Source: CAD feature listing. Evaluate the final solid. Frame: model axes, mm. Face numbers are marked on the shaded views. A direction names the side the tool comes from. Give positions to 0.01 mm unless a question says otherwise; leave off trailing zeros. Loops run counter-clockwise (first coordinate to the right, second up) from the corner with the lowest first, then second, coordinate; pieces in that order, holes last. Notation, with made-up numbers: M 79,14.5 L 136,14.5 A15 ccw 136,27.5 Z; hole C -21.5,54 d9. An arc over 180 degrees is marked long. Write item = value, one per line.
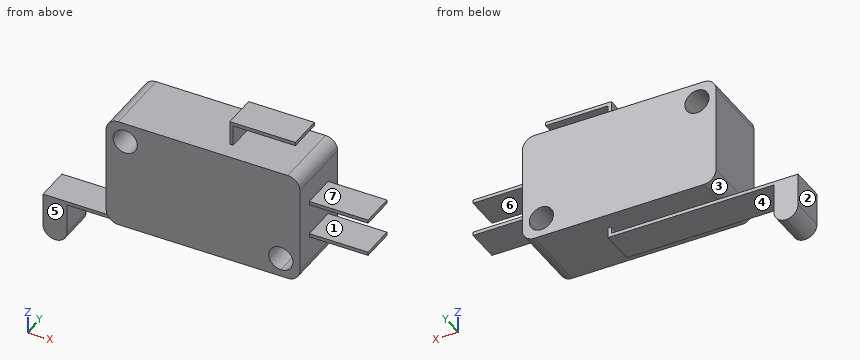
from build123d import *

# Parameters (mm, degrees)
SKETCH1_W           = 28
SKETCH1_H           = 16
BOSS_EXTRUDE1_DEPTH = 10
BOSS_EXTRUDE2_DEPTH = 1.5
SKETCH4_W           = 0.5
SKETCH4_H           = 5
BOSS_EXTRUDE3_DEPTH = 27
SKETCH6_W           = 3.5
SKETCH6_H           = 6
BOSS_EXTRUDE4_DEPTH = 5
FILLET1_R           = 1.75
BOSS_EXTRUDE5_DEPTH = 3.5
SKETCH8_W           = 0.5
SKETCH8_H           = 5
BOSS_EXTRUDE6_DEPTH = 9
BOSS_EXTRUDE7_DEPTH = 8.5
CUT_EXTRUDE1_DEPTH  = 45.547727215
CUT_EXTRUDE2_DEPTH  = 45.547727215
FILLET2_R           = 1.75


with BuildPart() as part:
    # Sketch1 → Boss-Extrude1 (new body)
    with BuildSketch(Plane(origin=(0, 0, 0), x_dir=(1, 0, 0), z_dir=(0, 1, 0))):
        with Locations((14, 8)):
            Rectangle(SKETCH1_W, SKETCH1_H)
    extrude(amount=BOSS_EXTRUDE1_DEPTH)

    # Sketch3 → Boss-Extrude2 (add)
    with BuildSketch(Plane(origin=(0, 0, -16), x_dir=(-1, 0, 0), z_dir=(0, 0, -1))):
        Polygon((-17, 2.5), (-17, 5), (-17, 7.5), (-16.5, 7.5), (-16.5, 2.5), align=None)
    extrude(amount=BOSS_EXTRUDE2_DEPTH)

    # Sketch4 → Boss-Extrude3 (add)
    with BuildSketch(Plane.ZY.offset(-16.5)):
        with Locations((-17.25, 5)):
            Rectangle(SKETCH4_W, SKETCH4_H)
    extrude(amount=BOSS_EXTRUDE3_DEPTH)

    # Sketch6 → Boss-Extrude4 (add)
    with BuildSketch(Plane.XZ.offset(-2.5)):
        with Locations((-8.75, -20.5)):
            Rectangle(SKETCH6_W, SKETCH6_H)
    extrude(amount=-BOSS_EXTRUDE4_DEPTH)

    # Fillet1
    fillet1_edges = [part.edges().sort_by_distance(p)[0] for p in [
        (-7, 5, -23.5),
        (-10.5, 5, -23.5),
    ]]
    fillet(fillet1_edges, radius=FILLET1_R - 0.0001)  # a hair under: the kernel refuses the full size

    # Sketch7 → Boss-Extrude5 (add)
    with BuildSketch(Plane.XY):
        Polygon((16.5, 2.5), (17, 2.5), (17, 5), (17, 7.5), (16.5, 7.5), align=None)
    extrude(amount=BOSS_EXTRUDE5_DEPTH)

    # Sketch8 → Boss-Extrude6 (add)
    with BuildSketch(Plane(origin=(17, 0, 0), x_dir=(0, 0, -1), z_dir=(1, 0, 0))):
        with Locations((-3.25, 5)):
            Rectangle(SKETCH8_W, SKETCH8_H)
    extrude(amount=BOSS_EXTRUDE6_DEPTH)

    # Sketch9 → Boss-Extrude7 (add)
    with BuildSketch(Plane(origin=(28, 0, 0), x_dir=(0, 0, -1), z_dir=(1, 0, 0))):
        Polygon((10, 2.5), (10.5, 2.5), (10.5, 5), (10.5, 7.5), (10, 7.5), align=None)
        Polygon((5, 5), (5, 7.5), (5.5, 7.5), (5.5, 2.5), (5, 2.5), align=None)
    extrude(amount=BOSS_EXTRUDE7_DEPTH)

    # Sketch10 → Cut-Extrude1 (cut, through all)
    with BuildSketch(Plane(origin=(0, 10, 0), x_dir=(1, 0, 0), z_dir=(0, 1, 0))):
        with BuildLine():
            ThreePointArc((25.25, 15), (24.012563133, 12.012563133), (27, 13.25))
            Line((27, 13.25), (25.25, 13.25))
            Line((25.25, 13.25), (25.25, 15))
        make_face()
        with BuildLine():
            Line((25.25, 13.25), (27, 13.25))
            ThreePointArc((27, 13.25), (26.487436867, 14.487436867), (25.25, 15))
            Line((25.25, 15), (25.25, 13.25))
        make_face()
    extrude(amount=-CUT_EXTRUDE1_DEPTH, mode=Mode.SUBTRACT)

    # Sketch11 → Cut-Extrude2 (cut, through all)
    with BuildSketch(Plane(origin=(0, 10, 0), x_dir=(1, 0, 0), z_dir=(0, 1, 0))):
        with BuildLine():
            ThreePointArc((4.5, 2.75), (2.75, 4.5), (1, 2.75))
            Line((1, 2.75), (2.75, 2.75))
            Line((2.75, 2.75), (2.75, 1))
            ThreePointArc((2.75, 1), (3.987436867, 1.512563133), (4.5, 2.75))
        make_face()
        with BuildLine():
            Line((2.75, 2.75), (1, 2.75))
            ThreePointArc((1, 2.75), (1.512563133, 1.512563133), (2.75, 1))
            Line((2.75, 1), (2.75, 2.75))
        make_face()
    extrude(amount=-CUT_EXTRUDE2_DEPTH, mode=Mode.SUBTRACT)

    # Fillet2
    fillet2_edges = [part.edges().sort_by_distance(p)[0] for p in [
        (0, 5, -16),
        (28, 5, -16),
        (28, 5, 0),
        (0, 5, 0),
    ]]
    fillet(fillet2_edges, radius=FILLET2_R)


solid = part.part
1. Pull-direction query (Z, two-part tool) for the marked faces 1, 2, 3 and 4; classes: +Z half, -Z half, draft (parallel to the pull), parting line (faces both ways), or undercut.
Derived:
face_1 = undercut
face_2 = draft
face_3 = undercut
face_4 = -Z half
2. Material intervals for probe 1 along Z at (x, y) = (25.25, 5.75); probe 2 along X at (y, z) = (7.25, -13.25); probe 3 along Z at (x, y) = (25.25, 7.75), sorted ascending. Write a range as from..to.
Derived:
probe_1 = -16..-15, -11.5..0, 3..3.5
probe_2 = 0..23.5, 27..28
probe_3 = -16..-15, -11.5..0
3. Reachability of the marked faces 5, 6 and 7 from +Z, -Z, +X, -X, +Y, -Y: full face, straight path, thin tool, end or side. Return the list, or none.
Derived:
face_5 = -Z, +X, -X, -Y
face_6 = +X, +Y, -Y
face_7 = +Z, +X, +Y, -Y
4. Cut plane A-A, the plane x = 13. Return the cut outline in (y, z).
Derived:
outline = M 0,-16 L 10,-16 L 10,0 L 0,0 Z; M 2.5,-17.5 L 7.5,-17.5 L 7.5,-17 L 2.5,-17 Z
5. First-contact query: pin 1 Ø0.6 at (x, z) = (31, -5.5) entering from +Y; pin 2 Ø0.6 at (x, z) = (33, -5) entering from -Y; pin 3 Ø1.5 at (x, y) = (31.5, 5) entering from -Z; pin 4 Ø4 at (x, z) = (20.5, 1.5) entering from +Y. Flat tips, straight axial feed; report the tip coordinate or a pass-through.
Derived:
pin_1 = 7.5
pin_2 = 2.5
pin_3 = -10.5
pin_4 = 10
6. Cut plane C-C, the plane x = 32. Return the cut outline in (y, z), then the cut area to 3 significant figures.
Derived:
outline = M 2.5,-10.5 L 7.5,-10.5 L 7.5,-10 L 2.5,-10 Z; M 2.5,-5.5 L 7.5,-5.5 L 7.5,-5 L 2.5,-5 Z
area = 5.00 mm²
7. Cut plane D-D, the plane z = -20.75. Return the cut outline in (x, y), then the cut area to 3 significant figures.
Derived:
outline = M -10.5,2.5 L -7,2.5 L -7,7.5 L -10.5,7.5 Z
area = 17.5 mm²
8. Cut plane B-B, the plane y = 6.75. Count the separate pieces of the cut face and the enclosed holes in it, then the cut area to 3 significant figures.
Derived:
separate_pieces = 1
enclosed_holes = 2
area = 475 mm²
